The drawing under review shows one solid part. Ordinate dimensions are in mm from its lowest x, y, z. A direction names the side the tool comes from. Coordinates: 2 decimals unless noted, no trailing zeros. Write each loop counter-clockwise with the first axis right and the second up, starting at its lowest first coordinate (ties: lowest second). Pieces come first, ordered by that corner, then holes.
Q1. Take a section at D-D (z = 43). Give the boundary of the cut face in (x, y), and give its area (3 significant figures).
Q2. Take a section at C-C (y = 4.25). Give the boundary of the cut face in (x, z), and give its area (4 significant figures).
Q3. Take a section at B-B (x = 21). Give the boundary of the cut face in (y, z), and give its area (3 significant figures).
Q4. Insertion check: pin 1 (2 mm diameter, centred on x = 38, y = 4.5, fed in from +Z); pin 2 (1.5 mm diameter, centred on x = 4.25, y = 37.75, fed in from +Z). Each pin has a flat end and moves straight along its axis. Give the tip position at first contact, or say it passes through.
Q5. Take a section at A-A (z = 36). Give the boundary of the cut face in (x, y), and give its area (3 significant figures).
Q6. For probe 1 along Y at (x, z) = (37.75, 37.7); probe 2 along Y at (x, z) = (37, 36); probe 3 along X at (y, z) = (4, 38), list the stretches that pass through material, from the lowest coordinate up.
Q7. Machinability: for the marked faces 1 and 2, which of the approach directions +Z, -Z, +X, -X, +Y, -Y give a long, thin tool a straight path to every point of the face, cutting with its end or side? Answer none if there is none.
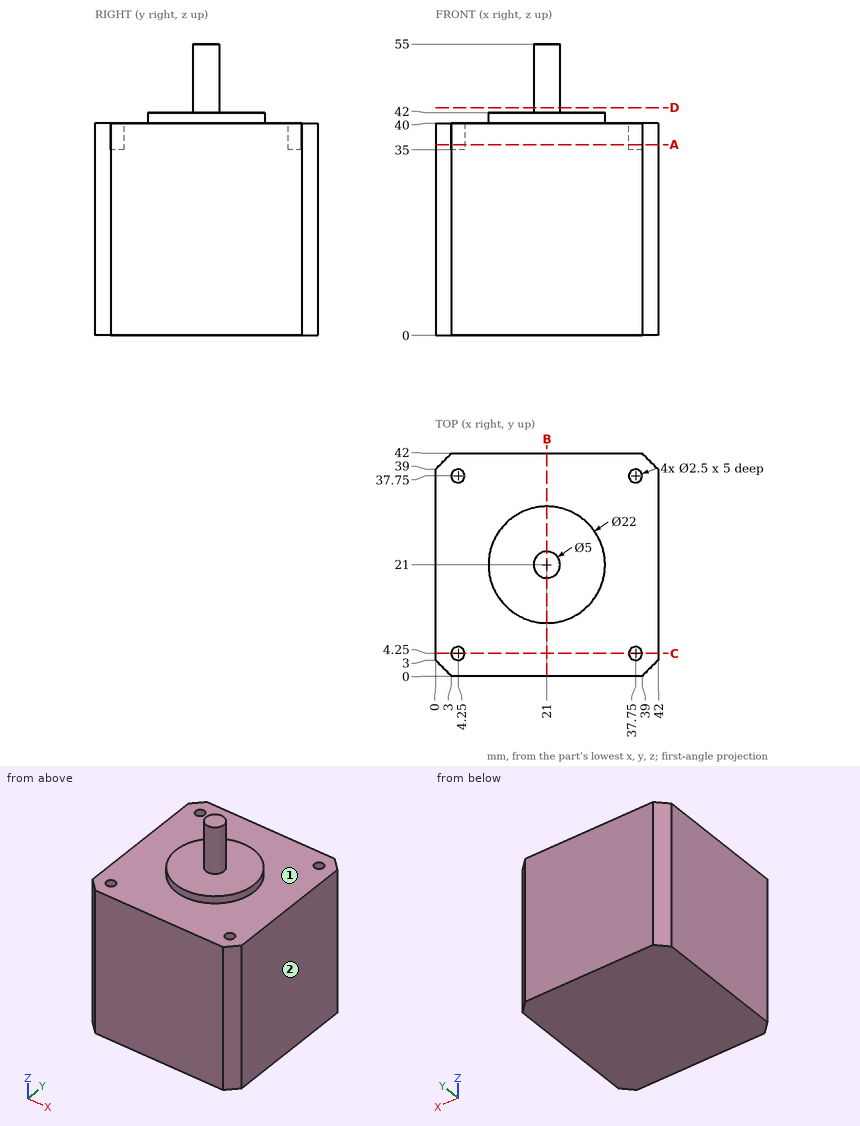
Response:
1. outline: circle Ø5 at (21, 21)
1. area: 19.6 mm2
2. outline: (0, 0) - (42, 0) - (42, 40) - (39, 40) - (39, 35) - (36.5, 35) - (36.5, 40) - (5.5, 40) - (5.5, 35) - (3, 35) - (3, 40) - (0, 40) - close
2. area: 1,655 mm2
3. outline: (0, 0) - (42, 0) - (42, 40) - (32, 40) - (32, 42) - (23.5, 42) - (23.5, 55) - (18.5, 55) - (18.5, 42) - (10, 42) - (10, 40) - (0, 40) - close
3. area: 1,790 mm2
4. pin 1: stops at z = 40
4. pin 2: stops at z = 35
5. outline: (0, 3) - (3, 0) - (39, 0) - (42, 3) - (42, 39) - (39, 42) - (3, 42) - (0, 39) - close; hole circle Ø2.5 at (4.25, 4.25); hole circle Ø2.5 at (4.25, 37.75); hole circle Ø2.5 at (37.75, 4.25); hole circle Ø2.5 at (37.75, 37.75)
5. area: 1,730 mm2
6. probe 1: y = 0 to 3, 5.5 to 36.5, 39 to 42
6. probe 2: y = 0 to 3.25, 5.25 to 36.75, 38.75 to 42
6. probe 3: x = 0 to 3.03, 5.47 to 36.53, 38.97 to 42
7. face 1: +Z
7. face 2: +Z, -Z, +X, +Y, -Y
